Verification items for the finished model (mm, model axes). Face numbers are marked on the shaded views. A direction names the side the tool comes from. Coordinates: 2 decimals unless noted, no trailing zeros. Loops run counter-clockwise (first coordinate to the right, second up) from the corner with the lowest first, then second, coordinate; pieces in that order, holes last.
Q1. Access from +Z, -Z, +X, -X, +Y, -Y to the whole of each face (thin tool, end or side, straight path). Record for the marked faces 1 and 2.
Q2. Sectioned sample at B-B (x = -41.5). Enter the section's corners in (y, z), then the cut area to 3 significant figures.
Q3. Sectioned sample at A-A (y = -26.5). Enter the section's corners in (x, z).
Q4. Sectioned sample at C-C (z = 16.75). Enter the section's corners in (x, y).
Q5. Material ranges on probe 1 along X at (y, z) = (23.5, 19), recorded low to high.
Q6. Go/stop test with flat-tipped pins: P1, Ø0.8, axis at x = 43, z = 0.5, coming from the -Y side; P2, Ø3, axis at x = 42.5, y = 0.5, coming from the +Z side; P3, Ø4, axis at y = 23, z = 10, coming from the -X side. Record where each tip stops, or that it passes through.
```python
from build123d import *

# Parameters (mm, degrees)
CROQUIS1_W              = 80
CROQUIS1_H              = 84
SALIENTE_EXTRUIR1_DEPTH = 25
CROQUIS4_W              = 10
CROQUIS4_H              = 84
SALIENTE_EXTRUIR3_DEPTH = 1
CROQUIS11_W             = 10
CROQUIS11_H             = 10
CORTAR_EXTRUIR1_DEPTH   = 1
CROQUIS8_W              = 10
CROQUIS8_H              = 10
CORTAR_EXTRUIR2_DEPTH   = 1


with BuildPart() as part:
    # Croquis1 → Saliente-Extruir1 (new body)
    with BuildSketch(Plane.XY):
        Rectangle(CROQUIS1_W, CROQUIS1_H)
    extrude(amount=SALIENTE_EXTRUIR1_DEPTH)

    # Croquis4 → Saliente-Extruir3 (add)
    with BuildSketch(Plane(origin=(0, 0, 0), x_dir=(-1, 0, 0), z_dir=(0, 0, -1))):
        with Locations((-45, 0)):
            Rectangle(CROQUIS4_W, CROQUIS4_H)
        with Locations((45, 0)):
            Rectangle(CROQUIS4_W, CROQUIS4_H)
    extrude(amount=-SALIENTE_EXTRUIR3_DEPTH)

    # Croquis11 → Cortar-Extruir1 (cut)
    with BuildSketch(Plane.XY.offset(1)):
        with Locations((-45, 37)):
            Rectangle(CROQUIS11_W, CROQUIS11_H)
        with Locations((-45, -37)):
            Rectangle(CROQUIS11_W, CROQUIS11_H)
    extrude(amount=-CORTAR_EXTRUIR1_DEPTH, mode=Mode.SUBTRACT)

    # Croquis8 → Cortar-Extruir2 (cut)
    with BuildSketch(Plane.XY.offset(1)):
        with Locations((45, 37)):
            Rectangle(CROQUIS8_W, CROQUIS8_H)
        with Locations((45, -37)):
            Rectangle(CROQUIS8_W, CROQUIS8_H)
    extrude(amount=-CORTAR_EXTRUIR2_DEPTH, mode=Mode.SUBTRACT)


solid = part.part
```
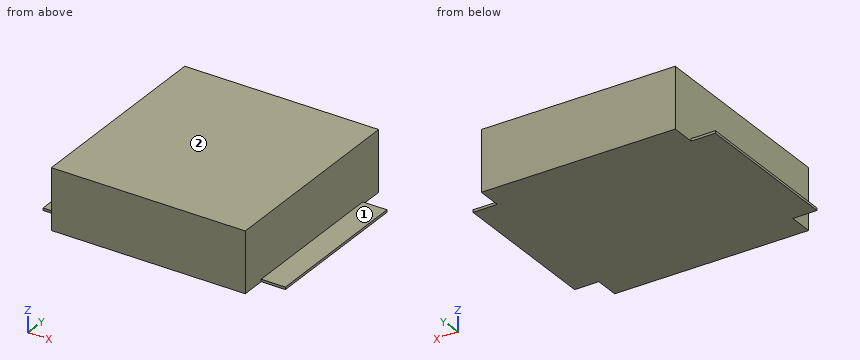
Geometry check:
1. face 1: +Z, +X, +Y, -Y
1. face 2: +Z, +X, -X, +Y, -Y
2. outline: (-32, 0) - (32, 0) - (32, 1) - (-32, 1) - close
2. area: 64.0 mm2
3. outline: (-50, 0) - (50, 0) - (50, 1) - (40, 1) - (40, 25) - (-40, 25) - (-40, 1) - (-50, 1) - close
4. outline: (-40, -42) - (40, -42) - (40, 42) - (-40, 42) - close
5. probe 1: x = -40 to 40
6. P1: stops at y = -32
6. P2: stops at z = 1
6. P3: stops at x = -40
